Drawing for the job (mm, zero at the part's lowest x, y, z). Give positions to 0.01 mm unless a question says otherwise; leave off trailing zeros. Order: outer loops, then holes, each group sorted by start corner. A loop starts at its lowest first (then second) coordinate and runs counter-clockwise, first axis right, second up. Notation, with made-up numbers: (53.5, 12) -> (67.5, 12) arc R20 cw to (67.5, 25) -> close; hole circle Ø10 at (29, 3). An arc over 180 degrees is marked (long way). One line per item, written item: value. Start each with the question number.
(1) Saw through at A-A on x = 60. Give the cut face in (y, z) (3 decimals), plus the area to 3 significant figures.
(2) Probe line 1 (Z direction, x = 60, y = 7.25); line 2 (X direction, y = 15.25, z = 2.75); line 3 (Y direction, x = 60, z = 0.6) (3 decimals). List the from-to ranges inside material, lowest first.
(3) Saw through at B-B on y = 16.5. Give the cut face in (x, z), plus the area to 3 significant figures.
(4) Pin check, flat tip, straight feed: pin 1 (3 mm diameter, centred on x = 60, y = 9.525, fed in from +Z). Stop position of the tip, or through.
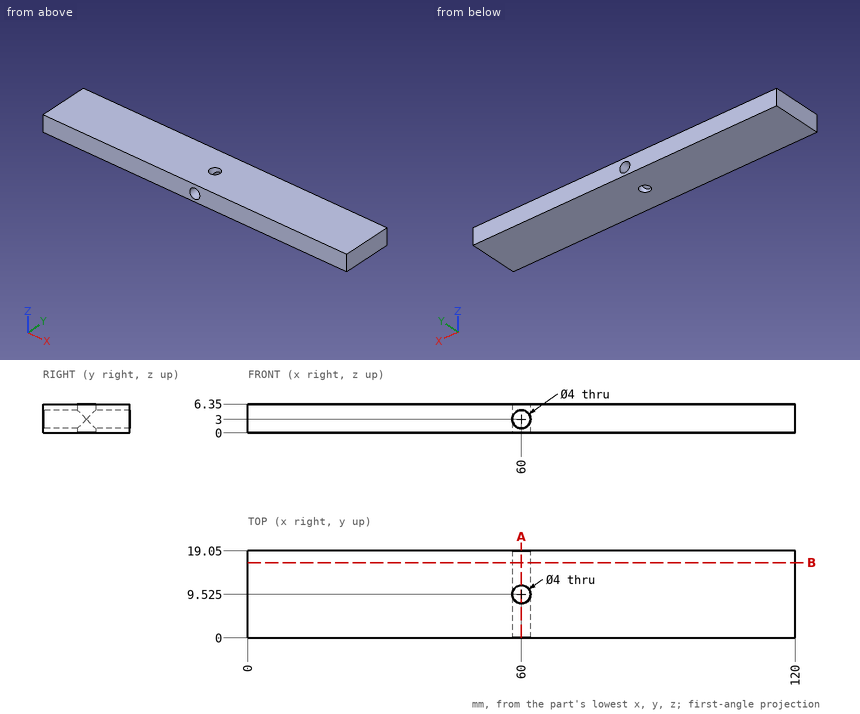
Results below:
1. outline: (0, 0) -> (7.525, 0) -> (7.525, 1) -> (0, 1) -> close; (0, 5) -> (7.525, 5) -> (7.525, 6.35) -> (0, 6.35) -> close; (11.525, 0) -> (19.05, 0) -> (19.05, 1) -> (11.525, 1) -> close; (11.525, 5) -> (19.05, 5) -> (19.05, 6.35) -> (11.525, 6.35) -> close
1. area: 35.4 mm²
2. line 1: z = 0 to 1, 5 to 6.35
2. line 2: x = 0 to 58.02, 61.98 to 120
2. line 3: y = 0 to 7.525, 11.525 to 19.05
3. outline: (0, 0) -> (120, 0) -> (120, 6.35) -> (0, 6.35) -> close; hole circle Ø4 at (60, 3)
3. area: 749 mm²
4. pin 1: passes through
